```python
from build123d import *

# Parameters (mm, degrees)
SKETCH_1_W               = 50
SKETCH_1_H               = 40
EXTRUDE_1_DEPTH          = 4
SKETCH_2_R               = 12.5
EXTRUDE_2_DEPTH          = 25
SKETCH_3_W               = 10
SKETCH_3_H               = 20
CUT_EXTRUDE_1_DEPTH      = 20
SKETCH_4_R               = 4
CUT_EXTRUDE_2_DEPTH      = 26
CUT_EXTRUDE_2_DEPTH_BACK = 26
SKETCH_5_R               = 3
CUT_EXTRUDE_3_DEPTH      = 10


with BuildPart() as part:
    # 草图1 → 凸台-拉伸1 (new body)
    with BuildSketch(Plane(origin=(0, 0, 0), x_dir=(1, 0, 0), z_dir=(0, 1, 0))):
        Rectangle(SKETCH_1_W, SKETCH_1_H)
    extrude(amount=EXTRUDE_1_DEPTH)

    # 草图2 → 凸台-拉伸2 (add)
    with BuildSketch(Plane(origin=(0, 4, 0), x_dir=(1, 0, 0), z_dir=(0, 1, 0))):
        Circle(SKETCH_2_R)
    extrude(amount=EXTRUDE_2_DEPTH)

    # 草图3 → 切除-拉伸1 (cut, symmetric)
    with BuildSketch(Plane.XY):
        with Locations((0, 19)):
            Rectangle(SKETCH_3_W, SKETCH_3_H)
    extrude(amount=CUT_EXTRUDE_1_DEPTH, both=True, mode=Mode.SUBTRACT)

    # 草图4 → 切除-拉伸2 (cut, two sides)
    with BuildSketch(Plane(origin=(0, 0, 0), x_dir=(0, 0, -1), z_dir=(1, 0, 0))) as cut_extrude_2_sk:
        with Locations((0, 19)):
            Circle(SKETCH_4_R)
    extrude(amount=CUT_EXTRUDE_2_DEPTH, mode=Mode.SUBTRACT)
    extrude(cut_extrude_2_sk.sketch, amount=-CUT_EXTRUDE_2_DEPTH_BACK, mode=Mode.SUBTRACT)

    # 草图5 → 切除-拉伸3 (cut)
    with BuildSketch(Plane(origin=(0, 4, 0), x_dir=(1, 0, 0), z_dir=(0, 1, 0))):
        with Locations((-20, 0)):
            Circle(SKETCH_5_R)
        with Locations((20, 0)):
            Circle(SKETCH_5_R)
    extrude(amount=-CUT_EXTRUDE_3_DEPTH, mode=Mode.SUBTRACT)


solid = part.part
```
Source: CAD feature listing. Evaluate the final solid. Frame: model axes, mm. A direction names the side the tool comes from. Round coordinates to 2 decimals unless told otherwise and drop trailing zeros. Order: outer loops, then holes, each group sorted by start corner. A loop starts at its lowest first (then second) coordinate and runs counter-clockwise, first axis right, second up. Notation, with made-up numbers: (13.5, 41.25) -> (18.5, 41.25) arc R3 ccw to (18.5, 46.25) -> close; hole circle Ø6 at (-29, 77). An arc over 180 degrees is marked (long way). Use CSV: the item, a comma, the result in double quotes.
(1) Section A-A on x = 20. Return the cut outline in (y, z), and give its area (3 significant figures).
Report:
outline,"(0, -20) -> (4, -20) -> (4, -3) -> (0, -3) -> close; (0, 3) -> (4, 3) -> (4, 20) -> (0, 20) -> close"
area,"136 mm^2"
(2) Section D-D on y = 3.25. Return the cut outline in (x, z), and give its area (3 significant figures).
Report:
outline,"(-25, -20) -> (25, -20) -> (25, 20) -> (-25, 20) -> close; hole circle Ø6 at (-20, 0); hole circle Ø6 at (20, 0)"
area,"1,940 mm^2"
(3) Section B-B on y = 17.5. Return the cut outline in (x, z), and give its area (3 significant figures).
Report:
outline,"(-11.94, -3.71) arc R12.5 ccw to (-5, -11.46) -> (-5, -3.71) -> close; (-11.94, 3.71) -> (-5, 3.71) -> (-5, 11.46) arc R12.5 ccw to start; (5, -11.46) arc R12.5 ccw to (11.94, -3.71) -> (5, -3.71) -> close; (5, 3.71) -> (11.94, 3.71) arc R12.5 ccw to (5, 11.46) -> close"
area,"139 mm^2"
(4) Access query for faces 1 (the face through (0, 9, 0)), 2 (the face through (-23, 2, 0)), 3 (the face through (0, 4, -14)). Directions: +Z, -Z, +X, -X, +Y, -Y. A direction counts if a zero-diameter tool reaches every point of the face in a straight line with its end or side. Return the directions, or none.
Report:
face 1,"+Z, -Z, +Y"
face 2,"+Y, -Y"
face 3,"+Y"
(5) Section C-C on z = -2. Return the cut outline in (x, y).
Report:
outline,"(-25, 0) -> (-22.24, 0) -> (-22.24, 4) -> (-25, 4) -> close; (-17.76, 0) -> (17.76, 0) -> (17.76, 4) -> (12.34, 4) -> (12.34, 15.54) -> (5, 15.54) -> (5, 9) -> (-5, 9) -> (-5, 15.54) -> (-12.34, 15.54) -> (-12.34, 4) -> (-17.76, 4) -> close; (-12.34, 22.46) -> (-5, 22.46) -> (-5, 29) -> (-12.34, 29) -> close; (5, 22.46) -> (12.34, 22.46) -> (12.34, 29) -> (5, 29) -> close; (22.24, 0) -> (25, 0) -> (25, 4) -> (22.24, 4) -> close"
(6) First-contact query: pin 1 Ø1 at (x, z) = (-4, -14) entering from +Y; pin 2 Ø1.5 at (x, y) = (7, 21.5) entering from +Z; pin 3 Ø2 at (y, z) = (18, -1) entering from -X; pin 4 Ø2 at (y, z) = (8, 9) entering from -X. Flat tips, straight axial feed; report the tip coordinate or a pass-through.
Report:
pin 1,"y = 4"
pin 2,"z = 10.83"
pin 3,"through"
pin 4,"x = -9.6"
(7) Ray query, L1, parallel to X at y = 1.3, z = 0; L2, parallel to Z at x = -20, y = 2.7; L3, parallel to Y at x = 10.75, z = 0. Return the intervals inside material, ascending.
Report:
L1,"-25 to -23, -17 to 17, 23 to 25"
L2,"-20 to -3, 3 to 20"
L3,"0 to 15, 23 to 29"
(8) Pull-direction query (Y, two-part tool) for faces 4 (the face through (5, 14, 0)), 5 (the face through (0, 0, 0)), 6 (the face through (9, 19, 4)), 7 (the face through (8, 29, 0)); classes: +Y half, -Y half, draft (parallel to the pull), parting line (faces both ways), or undercut.
Report:
face 4,"draft"
face 5,"-Y half"
face 6,"undercut"
face 7,"+Y half"
